from build123d import *

# Parameters (mm, degrees)
F0_W     = 210
F0_H     = 160
F1_DEPTH = 5
F2_R     = 5
F3_DEPTH = 5


with BuildPart() as f1:
    # F0 (on Front) → F1 (new body)
    with BuildSketch(Plane.XZ):
        with Locations((-5, -20)):
            Rectangle(F0_W, F0_H)
    extrude(amount=F1_DEPTH)

    # F2 (on face) → F3 (join)
    with BuildSketch(Plane.XZ.offset(5)):
        Circle(F2_R)
        with Locations((0, -60)):
            Circle(F2_R)
        with Locations((54, -60)):
            Circle(F2_R)
        with Locations((-66, 0)):
            Circle(F2_R)
    extrude(amount=F3_DEPTH)


solid = f1.part
Design review of the part built by this model. Coordinates are the model's own, in mm. A direction names the side the tool comes from. Give positions to 0.01 mm unless a question says otherwise; leave off trailing zeros. Order: outer loops, then holes, each group sorted by start corner. A loop starts at its lowest first (then second) coordinate and runs counter-clockwise, first axis right, second up.
1. Mouldability with a two-part tool opening along Z and no side actions: class faces 1 (the flat face through (0, -10, 0)), 2 (the cylindrical face through (-0.651, -7.465, -55.043)), 3 (the flat face through (-6, -2, -100)) as +Z half, -Z half, draft (parallel to the pull), parting line (faces both ways), or undercut.
Solution:
face 1: draft
face 2: undercut
face 3: -Z half
2. For pin 1 Ø6 at (x, z) = (69.5, -31.5) entering from -Y; pin 2 Ø4 at (x, y) = (26.5, -8.5) entering from +Z, all flat-tipped, find the tip position at first contact; note any pin that passes through.
Solution:
pin 1: stops at y = -5
pin 2: passes through
3. Add section D-D, the plane x = 0. State the section outline as (y, z) points.
Solution:
outline: (-10, -65) - (-5, -65) - (-5, -100) - (0, -100) - (0, 60) - (-5, 60) - (-5, 5) - (-10, 5) - (-10, -5) - (-5, -5) - (-5, -55) - (-10, -55) - close
4. Add section B-B, the plane z = 0. State the section outline as (x, y) points, then the cut area to 3 significant figures.
Solution:
outline: (-110, -5) - (-71, -5) - (-71, -10) - (-61, -10) - (-61, -5) - (-5, -5) - (-5, -10) - (5, -10) - (5, -5) - (100, -5) - (100, 0) - (-110, 0) - close
area: 1,150 mm2
5. Add section C-C, the plane y = -7.75. State the section outline as (x, z) points.
Solution:
outline: circle Ø10 at (-66, 0); circle Ø10 at (0, -60); circle Ø10 at (0, 0); circle Ø10 at (54, -60)
6. Tool access review of faces 4 (the cylindrical face through (-71, -7, 0)), 5 (the flat face through (-6, -2, 60)): name each direction out of +Z, -Z, +X, -X, +Y, -Y from which nothing blocks a thin tool from reaching the whole face with its end or side.
Solution:
face 4: -Y
face 5: +Z, +X, -X, +Y, -Y
7. Add section A-A, the plane x = 54. State the section outline as (y, z) points.
Solution:
outline: (-10, -65) - (-5, -65) - (-5, -100) - (0, -100) - (0, 60) - (-5, 60) - (-5, -55) - (-10, -55) - close
8. To check wall thickness, follow L1, parallel to Y at x = 41, z = -28; L2, parallel to Z at x = 1.5, y = -5.25; L3, parallel to X at y = -8, z = 4. State the ranges of each line that lie inside material, in increasing order.
Solution:
L1: y = -5 to 0
L2: z = -64.77 to -55.23, -4.77 to 4.77
L3: x = -69 to -63, -3 to 3
